```python
from build123d import *

# Parameters (mm, degrees)
DODANIE_WYCI_GNI_CIE1_DEPTH = 5


with BuildPart() as part:
    # Szkic1 → Dodanie-wyciągnięcie1 (new body)
    with BuildSketch(Plane.XY):
        with BuildLine():
            Line((-0.951045555, 20.39370068), (-1.925922284, 17.39370068))
            ThreePointArc((-1.925922284, 17.39370068), (-2.737603138, 17.28454596), (-3.543288168, 17.13753509))
            Line((-3.543288168, 17.13753509), (-5.397502016, 19.689451162))
            ThreePointArc((-5.397502016, 19.689451162), (-6.515515156, 20.052693732), (-7.206498161, 19.101672684))
            Line((-7.206498161, 19.101672684), (-7.206610043, 15.947249659))
            ThreePointArc((-7.206610043, 15.947249659), (-7.944833745, 15.592614173), (-8.665656885, 15.203828161))
            Line((-8.665656885, 15.203828161), (-11.217704483, 17.05786098))
            ThreePointArc((-11.217704483, 17.05786098), (-12.393246293, 17.057840133), (-12.756528516, 15.939839877))
            Line((-12.756528516, 15.939839877), (-11.7818646, 12.93977073))
            ThreePointArc((-11.7818646, 12.93977073), (-12.374368671, 12.374368671), (-12.93977073, 11.7818646))
            Line((-12.93977073, 11.7818646), (-15.939839877, 12.756528516))
            ThreePointArc((-15.939839877, 12.756528516), (-17.057840133, 12.393246293), (-17.05786098, 11.217704483))
            Line((-17.05786098, 11.217704483), (-15.203828161, 8.665656885))
            ThreePointArc((-15.203828161, 8.665656885), (-15.592614173, 7.944833745), (-15.947249659, 7.206610043))
            Line((-15.947249659, 7.206610043), (-19.101672684, 7.206498161))
            ThreePointArc((-19.101672684, 7.206498161), (-20.052693732, 6.515515156), (-19.689451162, 5.397502016))
            Line((-19.689451162, 5.397502016), (-17.13753509, 3.543288168))
            ThreePointArc((-17.13753509, 3.543288168), (-17.28454596, 2.737603138), (-17.39370068, 1.925922284))
            Line((-17.39370068, 1.925922284), (-20.39370068, 0.951045555))
            ThreePointArc((-20.39370068, 0.951045555), (-21.084649954, 0), (-20.39370068, -0.951045555))
            Line((-20.39370068, -0.951045555), (-17.39370068, -1.925922284))
            ThreePointArc((-17.39370068, -1.925922284), (-17.28454596, -2.737603138), (-17.13753509, -3.543288168))
            Line((-17.13753509, -3.543288168), (-19.689451162, -5.397502016))
            ThreePointArc((-19.689451162, -5.397502016), (-20.052693732, -6.515515156), (-19.101672684, -7.206498161))
            Line((-19.101672684, -7.206498161), (-15.947249659, -7.206610043))
            ThreePointArc((-15.947249659, -7.206610043), (-15.592614173, -7.944833745), (-15.203828161, -8.665656885))
            Line((-15.203828161, -8.665656885), (-17.05786098, -11.217704483))
            ThreePointArc((-17.05786098, -11.217704483), (-17.057840133, -12.393246293), (-15.939839877, -12.756528516))
            Line((-15.939839877, -12.756528516), (-12.93977073, -11.7818646))
            ThreePointArc((-12.93977073, -11.7818646), (-12.374368671, -12.374368671), (-11.7818646, -12.93977073))
            Line((-11.7818646, -12.93977073), (-12.756528516, -15.939839877))
            ThreePointArc((-12.756528516, -15.939839877), (-12.393246293, -17.057840133), (-11.217704483, -17.05786098))
            Line((-11.217704483, -17.05786098), (-8.665656885, -15.203828161))
            ThreePointArc((-8.665656885, -15.203828161), (-7.944833745, -15.592614173), (-7.206610043, -15.947249659))
            Line((-7.206610043, -15.947249659), (-7.206498161, -19.101672684))
            ThreePointArc((-7.206498161, -19.101672684), (-6.515515156, -20.052693732), (-5.397502016, -19.689451162))
            Line((-5.397502016, -19.689451162), (-3.543288168, -17.13753509))
            ThreePointArc((-3.543288168, -17.13753509), (-2.737603138, -17.28454596), (-1.925922284, -17.39370068))
            Line((-1.925922284, -17.39370068), (-0.951045555, -20.39370068))
            ThreePointArc((-0.951045555, -20.39370068), (0, -21.084649954), (0.951045555, -20.39370068))
            Line((0.951045555, -20.39370068), (1.925922284, -17.39370068))
            ThreePointArc((1.925922284, -17.39370068), (2.737603138, -17.28454596), (3.543288168, -17.13753509))
            Line((3.543288168, -17.13753509), (5.397502016, -19.689451162))
            ThreePointArc((5.397502016, -19.689451162), (6.515515156, -20.052693732), (7.206498161, -19.101672684))
            Line((7.206498161, -19.101672684), (7.206610043, -15.947249659))
            ThreePointArc((7.206610043, -15.947249659), (7.944833745, -15.592614173), (8.665656885, -15.203828161))
            Line((8.665656885, -15.203828161), (11.217704483, -17.05786098))
            ThreePointArc((11.217704483, -17.05786098), (12.393246293, -17.057840133), (12.756528516, -15.939839877))
            Line((12.756528516, -15.939839877), (11.7818646, -12.93977073))
            ThreePointArc((11.7818646, -12.93977073), (12.374368671, -12.374368671), (12.93977073, -11.7818646))
            Line((12.93977073, -11.7818646), (15.939839877, -12.756528516))
            ThreePointArc((15.939839877, -12.756528516), (17.057840133, -12.393246293), (17.05786098, -11.217704483))
            Line((17.05786098, -11.217704483), (15.203828161, -8.665656885))
            ThreePointArc((15.203828161, -8.665656885), (15.592614173, -7.944833745), (15.947249659, -7.206610043))
            Line((15.947249659, -7.206610043), (19.101672684, -7.206498161))
            ThreePointArc((19.101672684, -7.206498161), (20.052693732, -6.515515156), (19.689451162, -5.397502016))
            Line((19.689451162, -5.397502016), (17.13753509, -3.543288168))
            ThreePointArc((17.13753509, -3.543288168), (17.28454596, -2.737603138), (17.39370068, -1.925922284))
            Line((17.39370068, -1.925922284), (20.39370068, -0.951045555))
            ThreePointArc((20.39370068, -0.951045555), (21.084649954, 0), (20.39370068, 0.951045555))
            Line((20.39370068, 0.951045555), (17.39370068, 1.925922284))
            ThreePointArc((17.39370068, 1.925922284), (17.28454596, 2.737603138), (17.13753509, 3.543288168))
            Line((17.13753509, 3.543288168), (19.689451162, 5.397502016))
            ThreePointArc((19.689451162, 5.397502016), (20.052693732, 6.515515156), (19.101672684, 7.206498161))
            Line((19.101672684, 7.206498161), (15.947249659, 7.206610043))
            ThreePointArc((15.947249659, 7.206610043), (15.592614173, 7.944833745), (15.203828161, 8.665656885))
            Line((15.203828161, 8.665656885), (17.05786098, 11.217704483))
            ThreePointArc((17.05786098, 11.217704483), (17.057840133, 12.393246293), (15.939839877, 12.756528516))
            Line((15.939839877, 12.756528516), (12.93977073, 11.7818646))
            ThreePointArc((12.93977073, 11.7818646), (12.374368671, 12.374368671), (11.7818646, 12.93977073))
            Line((11.7818646, 12.93977073), (12.756528516, 15.939839877))
            ThreePointArc((12.756528516, 15.939839877), (12.393246293, 17.057840133), (11.217704483, 17.05786098))
            Line((11.217704483, 17.05786098), (8.665656885, 15.203828161))
            ThreePointArc((8.665656885, 15.203828161), (7.944833745, 15.592614173), (7.206610043, 15.947249659))
            Line((7.206610043, 15.947249659), (7.206498161, 19.101672684))
            ThreePointArc((7.206498161, 19.101672684), (6.515515156, 20.052693732), (5.397502016, 19.689451162))
            Line((5.397502016, 19.689451162), (3.543288168, 17.13753509))
            ThreePointArc((3.543288168, 17.13753509), (2.737603138, 17.28454596), (1.925922284, 17.39370068))
            Line((1.925922284, 17.39370068), (0.951045555, 20.39370068))
            ThreePointArc((0.951045555, 20.39370068), (0, 21.084649954), (-0.951045555, 20.39370068))
        make_face()
        with BuildLine():
            Line((-2, 1.5), (-2, -1.5))
            ThreePointArc((-2, -1.5), (2.5, 0), (-2, 1.5))
        make_face(mode=Mode.SUBTRACT)
    extrude(amount=DODANIE_WYCI_GNI_CIE1_DEPTH)


solid = part.part
```
Work out the finished part from the listing and answer in its coordinate system (mm). A direction names the side the tool comes from. Give positions to 0.01 mm unless a question says otherwise; leave off trailing zeros. Order: outer loops, then holes, each group sorted by start corner. A loop starts at its lowest first (then second) coordinate and runs counter-clockwise, first axis right, second up.
1. For faces 1 (the flat face through (0, 5, 5)), 2 (the cylindrical face through (-2.726, 17.286, 2.465)), 3 (the flat face through (-4.48, -18.43, 2.46)), 4 (the flat face through (18.915, 1.432, 2.465)), 5 (the cylindrical face through (-15.6, -7.93, 2.46)), determine the directions among +Z, -Z, +X, -X, +Y, -Y from which every point of the face is accessible in a straight line to the end or side of a thin tool.
Result sheet:
face 1: +Z, +X, -X, +Y, -Y
face 2: +Z, -Z, +Y
face 3: +Z, -Z, -Y
face 4: +Z, -Z, +X
face 5: +Z, -Z, -X
2. Straight lines are drawn through the part: L1, parallel to X at y = -2, z = 1.75; L2, parallel to Y at x = 18.5, z = 0.3; L3, parallel to Y at x = -16, z = 3.45. For each, find the intervals that lie inside material, in ascending order.
Result sheet:
L1: x = -17.39 to -1.5, 1.5 to 17.39
L2: y = -7.21 to -4.53, -1.57 to 1.57, 4.53 to 7.21
L3: y = -12.77 to -9.76, -7.21 to 7.21, 9.76 to 12.77
3. Section D-D, the plane x = -10.5 is taken. Determine the outline of the cut face in (y, z), and give its area (3 significant figures).
Result sheet:
outline: (-16.54, 0) - (16.54, 0) - (16.54, 5) - (-16.54, 5) - close
area: 165 mm2
4. The mould has two halves that part along X. Classify faces 6 (the cylindrical face through (-20.058, -6.499, 2.465)), 7 (the cylindrical face through (12.37, -12.38, 2.46)), 8 (the cylindrical face through (6.532, 20.047, 2.465)), 9 (the flat face through (18.873, -1.445, 2.465)): released by +X, released by -X, zero draft, split by the parting line, or undercut.
Result sheet:
face 6: released by -X
face 7: undercut
face 8: undercut
face 9: released by +X
5. Section C-C, the plane y = 8 is taken. Determine the outline of the cut face in (x, z).
Result sheet:
outline: (-15.56, 0) - (15.56, 0) - (15.56, 5) - (-15.56, 5) - close
6. Section A-A, the plane y = 0 is taken. Determine the outline of the cut face in (x, z).
Result sheet:
outline: (-21.08, 0) - (-2, 0) - (-2, 5) - (-21.08, 5) - close; (2.5, 0) - (21.08, 0) - (21.08, 5) - (2.5, 5) - close
7. Section B-B, the plane x = 0 is taken. Determine the outline of the cut face in (y, z), and give its area (3 significant figures).
Result sheet:
outline: (-21.08, 0) - (-2.5, 0) - (-2.5, 5) - (-21.08, 5) - close; (2.5, 0) - (21.08, 0) - (21.08, 5) - (2.5, 5) - close
area: 186 mm2
8. Each of these flat-tipped pins is pushed along its axis until it touches: P1, Ø1.6, axis at y = 17.5, z = 3, coming from the -X side; P2, Ø1.6, axis at x = 17, z = 3, coming from the +Y side. Where does it stop, or does it pass through?
Result sheet:
P1: stops at x = -12.7
P2: stops at y = 12.81
